Autodesk Inventor part; units mm, degrees
ref_plane "YZ Plane" through (0, 0, 0) normal (1, 0, 0) x (0, 1, 0)
ref_plane "XZ Plane" through (0, 0, 0) normal (0, 1, 0) x (-1, 0, 0)
ref_plane "XY Plane" through (0, 0, 0) normal (0, 0, 1) x (1, 0, 0)
sketch "Sketch1" plane through (0, 0, 0) normal (0, 0, 1) x (1, 0, 0)
  arc A0 (-37.5, -13.9194) -> (37.5, -13.9194) centre (0, 0) ccw
  line L0 (-37.5, -13.9194) -> (-37.5, 21.0806)
  line L1 (37.5, -13.9194) -> (37.5, 21.0806)
  arc A1 (-42.5, -14.7902) -> (42.5, -14.7902) centre (0, 0) ccw
  line L2 (-42.5, -14.7902) -> (-42.5, 21.0806)
  line L3 (42.5, -14.7902) -> (42.5, 21.0806)
  line L4 (77.5, 21.0806) -> (77.5, -19.8431)
  line L5 (-77.5, -19.8431) -> (-77.5, 21.0806)
  line L6 (82.5, 21.0806) -> (82.5, -20.4634)
  line L7 (-82.5, -20.4634) -> (-82.5, 21.0806)
  line L8 (17.5, -113.0625) -> (17.5, -78.0625)
  line L9 (-17.5, -113.0625) -> (-17.5, -78.0625)
  line L10 (22.5, -81.968) -> (22.5, -108.0625)
  line L11 (-22.5, -108.0625) -> (-22.5, -81.968)
  line L12 (22.5, -108.0625) -> (17.5, -108.0625)
  arc A2 (-77.5, -19.8431) -> (-17.5, -78.0625) centre (0, 0) ccw
  arc A3 (17.5, -78.0625) -> (77.5, -19.8431) centre (0, 0) ccw
  arc A4 (-82.5, -20.4634) -> (-22.5, -81.968) centre (0, 0) ccw
  arc A5 (22.5, -81.968) -> (82.5, -20.4634) centre (0, 0) ccw
  line L13 (-17.5, -113.0625) -> (-17.5, -108.0625)
  line L14 (17.5, -113.0625) -> (17.5, -108.0625)
  line L15 (-82.5, 21.0806) -> (-77.5, 21.0806)
  line L16 (-42.5, 21.0806) -> (-37.5, 21.0806)
  line L17 (37.5, 21.0806) -> (42.5, 21.0806)
  line L18 (77.5, 21.0806) -> (82.5, 21.0806)
  line L19 (-22.5, -13.9194) -> (-17.5, -13.9194)
  line L20 (17.5, -13.9194) -> (22.5, -13.9194)
  line L21 (-77.5, 21.0806) -> (82.5, 21.0806)
  line L22 (1.8649, -108.0625) -> (17.5, -108.0625)
  line L23 (22.5, -108.0625) -> (22.5, -143.0625)
  line L24 (17.5, -143.0625) -> (17.5, -108.0625)
  line L25 (-17.5, -108.0625) -> (-17.5, -113.0625)
  line L26 (22.5, -178.0625) -> (22.5, -178.0625)
  line L27 (-17.5, -183.0625) -> (-287.4597, -183.0625)
  line L28 (-17.5, -178.0625) -> (-287.099, -178.0625)
  line L29 (-287.4597, -138.0625) -> (-47.5, -138.0625)
  line L30 (-22.5, -113.0625) -> (-22.5, -108.0625)
  line L31 (-287.4597, -183.0625) -> (-287.4597, -138.0625)
  line L32 (-17.5, -78.0625) -> (17.5, -78.0625)
  line L33 (-243.2803, -138.0625) -> (-242.0268, -183.0625)
  arc A6 (-17.5, -178.0625) -> (17.5, -143.0625) centre (-17.5, -143.0625) ccw
  arc A7 (-17.5, -183.0625) -> (22.5, -143.0625) centre (-17.5, -143.0625) ccw
  arc A8 (-47.5, -143.0625) -> (-17.5, -113.0625) centre (-47.5, -113.0625) ccw
  arc A9 (-47.5, -138.0625) -> (-22.5, -113.0625) centre (-47.5, -113.0625) ccw
  line L34 (-47.5, -143.0625) -> (-287.4597, -143.0625)
  line L35 (-22.5, -113.0625) -> (-22.5, -108.0625)
  point P0 (-42.5, 21.0806)
  point P1 (77.5, 21.0806)
  point P2 (42.5, 21.0806)
  point P3 (17.5, -162.4274)
  point P4 (-287.5, -178.0625)
  point P5 (37.5, 21.0806)
  point P6 (-243.1411, -143.0625)
  point P7 (-242.1661, -178.0625)
  dimension "d0" = 75
  dimension "d1" = 40
  dimension "d2" = 35
  dimension "d3" = 35
  dimension "d4" = 5
  dimension "d5" = 5
  dimension "d6" = 5
  dimension "d9" = 35
  dimension "d10" = 20
  dimension "d11" = 5
  dimension "d12" = 0
  dimension "d13" = 0
  dimension "d14" = 5
  dimension "d21" = 35
  dimension "d22" = 310
  dimension "d23" = 305
  dimension "d24" = 5
  dimension "d31" = 100
  dimension "d32" = 85
  dimension "d33" = 80
  dimension "d34" = 78.0625
  dimension "d37" = 5
extrude "Extrusion1" add sketch "Sketch1" along normal blind 20 contours A0 L1 L17 L3 A1 L2 L16 L0 | L5 A2 L9 A8 L34 L33 L29 A9 L30 L11 A4 L7 L15 | L18 L6 A5 L10 L12 L8 A3 L4 | L12 L23 A7 L27 L33 L28 A6 L24 L8
extrude "Extrusion2" add sketch "Sketch1" along normal blind 5 contours L2 A1 L3 L21 L4 A3 L32 A2 L5 | L18 L6 A5 L10 L12 L8 A3 L4 | L32 L8 L24 A6 L28 L33 L34 A8 L9
extrude "Extrusion3" cut sketch "Sketch1" along normal through all both and the other way through all contours L34 L31 L29 L33 | L33 L27 L31 L34
equation "\"d3\" = d2"
properties part number "storrageout"
For this review, take the finished solid that the model builds, in its own axes (mm). A direction names the side the tool comes from. Round coordinates to 2 decimals unless told otherwise and drop trailing zeros. Order: outer loops, then holes, each group sorted by start corner. A loop starts at its lowest first (then second) coordinate and runs counter-clockwise, first axis right, second up. Notation, with made-up numbers: M 10.5,9.25 L 31.5,9.25 A24 cw 31.5,41.25 Z; hole C 19,-14.75 d9. An arc over 180 degrees is marked long. Write each question's results on one line, items separated by ' | '. Start each with the question number.
1. Add section A-A (y = -6). State the section outline as (x, z) points.
2. Add section D-D (y = -32). State the section outline as (x, z) points.
3. Clearance check with flat-ended pins moving along their axes: pin 1 Ø6 at (y, z) = (-94.5, 9.5) entering from -X; pin 2 Ø6 at (y, z) = (-117.5, 9.5) entering from +X; pin 3 Ø7.5 at (y, z) = (8.5, 16) entering from -X. State where each tip first meets the part, or that it passes through.
4. To check wall thickness, follow L1, parallel to Y at x = -39.5, z = 15.5; L2, parallel to Y at x = -196, z = 8.75; L3, parallel to Y at x = -64.5, z = 10. State the ranges of each line that lie inside material, in increasing order. Write a range as [from, to].
5. Tool access review of faces 4 (the face through (-82.5, 0, 10)), 5 (the face through (0.779, -44.993, 12.395)), 6 (the face through (-42.5, 3, 12)), 7 (the face through (-144, -143.062, 12)): name each direction out of +Z, -Z, +X, -X, +Y, -Y from which nothing blocks a thin tool from reaching the whole face with its end or side.
6. Draft analysis for pull direction X (two halves, no side actions). For faces 1 (the face through (61.282, -58.902, 9.86)), 2 (the face through (42.5, 3, 12)), 3 (the face through (-22.5, -98, 10)), state which applies: pulls with the +X half, pulls with the -X half, needs draft (parallel to the pull), parting line crosses it, or undercut.
7. Add section C-C (y = -108). State the section outline as (x, z) points, then the cut area to 3 significant figures.
8. Add section B-B (x = -106). State the section outline as (y, z) points.
Output values:
1) outline: M -82.5,0 L -37.5,0 L -37.5,20 L -42.5,20 L -42.5,5 L -77.5,5 L -77.5,20 L -82.5,20 Z; M 37.5,0 L 82.5,0 L 82.5,20 L 77.5,20 L 77.5,5 L 42.5,5 L 42.5,20 L 37.5,20 Z
2) outline: M -78.75,0 L -24,0 L -24,20 L -31.64,20 L -31.64,5 L -73.32,5 L -73.32,20 L -78.75,20 Z; M 24,0 L 78.75,0 L 78.75,20 L 73.32,20 L 73.32,5 L 31.64,5 L 31.64,20 L 24,20 Z
3) pin 1: x = -22.5 | pin 2: x = 22.5 | pin 3: x = -82.5
4) L1: [-183.06, -178.06], [-141.98, -136.75], [-75.26, -69.57], [-21.56, 21.08] | L2: [-183.06, -178.06], [-143.06, -138.06] | L3: [-183.06, -178.06], [-143.06, -138.06], [-55.36, -47.33]
5) face 4: +Z, -Z, -X, +Y | face 5: +Z | face 6: +Z, +Y | face 7: +Z, -X
6) face 1: pulls with the +X half | face 2: undercut | face 3: pulls with the -X half
7) outline: M -22.5,0 L 22.5,0 L 22.5,20 L 17.5,20 L 17.5,5 L -17.5,5 L -17.5,20 L -22.5,20 Z | area: 375 mm^2
8) outline: M -183.06,0 L -138.06,0 L -138.06,20 L -143.06,20 L -143.06,5 L -178.06,5 L -178.06,20 L -183.06,20 Z
